Geometry check sheet. Reference: the model listing, model coordinates, mm. A direction names the side the tool comes from. Coordinates: 2 decimals unless noted, no trailing zeros. Order: outer loops, then holes, each group sorted by start corner. A loop starts at its lowest first (then second) coordinate and runs counter-clockwise, first axis right, second up. Notation, with made-up numbers: M 24.5,-4 L 33.5,-4 A22 cw 33.5,14 Z; hole C 52,57 d2. An arc over 180 degrees is marked long. One line per item, written item: value. Start each with the question number.
1) Sectioned sample at A-A, the plane z = 0. Enter the section's corners in (x, y).
2) Thickness scan on L1, parallel to Y at x = -0.2, z = -0.45; L2, parallel to X at y = 4.5, z = 0.2; L3, parallel to Y at x = -1.55, z = -0.4. Record the ranges inside material, lowest first. Write a range as from..to.
3) Sectioned sample at B-B, the plane y = -2.5. Enter the section's corners in (x, z), then the cut area to 3 significant figures.
4) Draft check along Z on faces 1 (the flat face through (0.75, 4, 0)), 2 (the flat face through (0, -5, 0)), 3 (the cylindrical face through (-1.9, 4.01, -0.08)). Enter one of: pulls with the +Z half, pulls with the -Z half, needs draft (parallel to the pull), parting line crosses it, or undercut.
5) Go/stop test with a flat-tipped pin: P1, Ø0.8, axis at x = 0, z = -0.5, coming from the +Y side. Record where the tip stops, or that it passes through.
6) Access from +Z, -Z, +X, -X, +Y, -Y to the whole of each face (thin tool, end or side, straight path). Record for faces 4 (the flat face through (1, 5, -1)), 5 (the flat face through (-0.75, 4, 0)), 6 (the cylindrical face through (0, -1, 1)).
Autodesk Inventor part; units mm, degrees
ref_plane "YZ Plane" through (0, 0, 0) normal (1, 0, 0) x (0, 1, 0)
ref_plane "XZ Plane" through (0, 0, 0) normal (0, 1, 0) x (-1, 0, 0)
ref_plane "XY Plane" through (0, 0, 0) normal (0, 0, 1) x (1, 0, 0)
sketch "Sketch1" plane through (0, 0, 0) normal (0, 0, 1) x (1, 0, 0)
  line L0 (0, 5) -> (0, -5)
  line L1 (0, -5) -> (0.75, -5)
  line L2 (0.75, -5) -> (1, -4.75)
  line L3 (1, -4.75) -> (1, 2.9)
  line L4 (1.1, 3) -> (1.65, 3)
  line L5 (1.9, 3.25) -> (1.9, 4.75)
  line L6 (1.65, 5) -> (0, 5)
  arc A0 (1.1, 3) -> (1, 2.9) centre (1.1, 2.9) ccw
  line L7 (1.65, 5) -> (1.9, 4.75)
  line L8 (1.65, 3) -> (1.9, 3.25)
  point P0 (0, 0)
  point P1 (1.9, 3)
  point P2 (1.9, 5)
  point P3 (0, 0)
  dimension "d0" = 3.8
  dimension "d1" = 2
  dimension "d3" = 2
  dimension "d4" = 2.2
  dimension "d5" = 135
  dimension "d6" = 0.25
  dimension "d7" = 8
  dimension "d18" = 0.25
revolve "Revolution1" add sketch "Sketch1" angle 360 about axis through (0, 5, 0) along (0, -1, 0)
sketch "Sketch2" plane through (0, 5, 0) normal (0, 1, 0) x (1, 0, 0)
  line L0 (0, -0.866) -> (-0.75, -0.433)
  line L1 (-0.75, -0.433) -> (-0.75, 0.433)
  line L2 (-0.75, 0.433) -> (0, 0.866)
  line L3 (0, 0.866) -> (0.75, 0.433)
  line L4 (0.75, 0.433) -> (0.75, -0.433)
  line L5 (0.75, -0.433) -> (0, -0.866)
  point P0 (0, 0)
  point P1 (0, 0)
  dimension "d11" = 1.5
extrude "Extrusion1" cut sketch "Sketch2" against normal blind 1.5
thread "Thread1"
sketch "Sketch3" plane through (0, 0, 0) normal (1, 0, 0) x (0, 1, 0)
  line L0 (5, 0.866) -> (5, 0.433)
  line L1 (5, 0.866) -> (4.5, 0.366)
  line L2 (4.5, 0.366) -> (5, 0.366)
  line L3 (5, 0.366) -> (5, 0.866)
  line L4 (-1, 0) -> (6, 0)
  point P0 (0, 0)
  dimension "d16" = 0.5
revolve "Revolution2" cut sketch "Sketch3" angle 360 about axis through (0, -10, 0) along (0, 1, 0)
properties part number "Bolt_M2x0.4_8mm_SH" material "Stainless Steel"
Final values:
1. outline: M -1.9,3.25 L -1.65,3 L -1.1,3 A0.1 cw -1,2.9 L -1,-4.75 L -0.75,-5 L 0.75,-5 L 1,-4.75 L 1,2.9 A0.1 cw 1.1,3 L 1.65,3 L 1.9,3.25 L 1.9,4.75 L 1.65,5 L 0.87,5 L 0.75,4.88 L 0.75,3.5 L -0.75,3.5 L -0.75,4.88 L -0.87,5 L -1.65,5 L -1.9,4.75 Z
2. L1: y = -5..3.5
2. L2: x = -1.89..-0.75, 0.75..1.89
2. L3: y = 3..5
3. outline: C 0,0 d2
3. area: 3.14 mm^2
4. face 1: undercut
4. face 2: needs draft
4. face 3: parting line crosses it
5. P1: stops at y = 5
6. face 4: +Z, -Z, +X, -X, +Y
6. face 5: +Y
6. face 6: -Y
